Check sheet for the modelled part. Datum: model origin and axes. Units: mm. Give positions to 0.01 mm unless a question says otherwise; leave off trailing zeros. Order: outer loops, then holes, each group sorted by start corner. A loop starts at its lowest first (then second) coordinate and runs counter-clockwise, first axis right, second up. Notation, with made-up numbers: (-8.5, 45) -> (2.5, 45) arc R16 cw to (2.5, 70) -> close; hole circle Ø3 at (14, 70.25). An arc over 180 degrees is marked (long way). One line per question, with ' | ' between items.
```python
from build123d import *

# Parameters (mm, degrees)
ESBO_O1_W                = 60
ESBO_O1_H                = 130
RESSALTO_EXTRUS_O1_DEPTH = 4
ESBO_O2_R                = 19
ESBO_O2_R_2              = 2.5
CORTE_EXTRUS_O1_DEPTH    = 72.700767081
FURO_COM_FOLGA_DE_M51_D  = 5.3


with BuildPart() as part:
    # Esboço1 → Ressalto-extrusão1 (new body)
    with BuildSketch(Plane(origin=(0, 0, 0), x_dir=(1, 0, 0), z_dir=(0, 1, 0))):
        Rectangle(ESBO_O1_W, ESBO_O1_H)
    extrude(amount=RESSALTO_EXTRUS_O1_DEPTH)

    # Esboço2 → Corte-extrusão1 (cut, through all)
    with BuildSketch(Plane(origin=(0, 4, 0), x_dir=(1, 0, 0), z_dir=(0, 1, 0))):
        with Locations(Location((0, 0, 0), (0, 0, 270))):
            Circle(ESBO_O2_R)
        with Locations(Location((-23.57, 23.57, 0), (0, 0, 270))):
            Circle(ESBO_O2_R_2)
        with Locations(Location((23.57, 23.57, 0), (0, 0, 270))):
            Circle(ESBO_O2_R_2)
        with Locations(Location((23.57, -23.57, 0), (0, 0, 270))):
            Circle(ESBO_O2_R_2)
        with Locations(Location((-23.57, -23.57, 0), (0, 0, 270))):
            Circle(ESBO_O2_R_2)
    extrude(amount=-CORTE_EXTRUS_O1_DEPTH, mode=Mode.SUBTRACT)

    # Furo com folga de M51 (through all)
    with Locations(Plane(origin=(0, 4, 0), x_dir=(1, 0, 0), z_dir=(0, 1, 0))):
        with Locations((-20, -50), (20, -50), (-20, 50), (20, 50)):
            Hole(FURO_COM_FOLGA_DE_M51_D / 2)


solid = part.part
```
Q1. Section check B-B (x = 0). Enter the section's corners in (y, z).
Result sheet:
outline: (0, -65) -> (4, -65) -> (4, -19) -> (0, -19) -> close; (0, 19) -> (4, 19) -> (4, 65) -> (0, 65) -> close
Q2. Thickness scan on line 1 (Z direction, x = 20, y = 2.85); line 2 (X direction, y = 2.95, z = 50); line 3 (X direction, y = 1.3, z = 23.57). Record the ranges inside material, lowest first.
Result sheet:
line 1: z = -65 to -52.65, -47.35 to 47.35, 52.65 to 65 | line 2: x = -30 to -22.65, -17.35 to 17.35, 22.65 to 30 | line 3: x = -30 to -26.07, -21.07 to 21.07, 26.07 to 30
Q3. Section check C-C (y = 3.1). Count the separate pieces of the cut face and the enclosed holes in it, and give its area (3 significant figures).
Result sheet:
separate pieces: 1 | enclosed holes: 9 | area: 6,500 mm2
Q4. Section check A-A (z = -50). Enter the section's corners in (x, y), and give its area (3 significant figures).
Result sheet:
outline: (-30, 0) -> (-22.65, 0) -> (-22.65, 4) -> (-30, 4) -> close; (-17.35, 0) -> (17.35, 0) -> (17.35, 4) -> (-17.35, 4) -> close; (22.65, 0) -> (30, 0) -> (30, 4) -> (22.65, 4) -> close | area: 198 mm2
Q5. Mould release check, pull along Z, two halves, no side actions. Record for faces 1 (the face through (-30, 2, 1)), 2 (the face through (0, 2, 65)), 3 (the face through (25.68, 2.03, -22.23)): pulls with the +Z half, pulls with the -Z half, needs draft (parallel to the pull), parting line crosses it, or undercut.
Result sheet:
face 1: needs draft | face 2: pulls with the +Z half | face 3: undercut
Q6. Section check D-D (z = -23.57). Enter the section's corners in (x, y).
Result sheet:
outline: (-30, 0) -> (-26.07, 0) -> (-26.07, 4) -> (-30, 4) -> close; (-21.07, 0) -> (21.07, 0) -> (21.07, 4) -> (-21.07, 4) -> close; (26.07, 0) -> (30, 0) -> (30, 4) -> (26.07, 4) -> close
Q7. Depth check by flat-ended pin: pin 1 Ø5 at (x, z) = (-20, 50) entering from +Y. Enter the tip coordinate at first touch or a pass-through.
Result sheet:
pin 1: passes through
